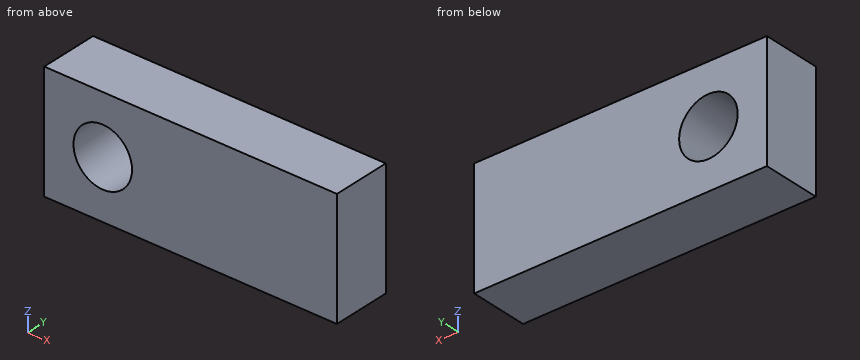
```python
from build123d import *

# Parameters (mm, degrees)
SKETCH2_W           = 127
SKETCH2_H           = 50.8
BOSS_EXTRUDE2_DEPTH = 25.4
CUT_EXTRUDE1_REACH  = 27.4
SKETCH3_R           = 12.7


with BuildPart() as part:
    # Sketch2 → Boss-Extrude2 (new body)
    with BuildSketch(Plane(origin=(0, 0, 0), x_dir=(1, 0, 0), z_dir=(0, 1, 0))):
        with Locations((63.5, 25.4)):
            Rectangle(SKETCH2_W, SKETCH2_H)
    extrude(amount=BOSS_EXTRUDE2_DEPTH)

    # Sketch3 → Cut-Extrude1 (cut, up to next)
    with BuildSketch(Plane.XZ, mode=Mode.PRIVATE) as cut_extrude1_sk1:
        with Locations((25.4, -25.4)):
            Circle(SKETCH3_R)
    cut_extrude1_tool1 = extrude(cut_extrude1_sk1.sketch, amount=-CUT_EXTRUDE1_REACH, mode=Mode.PRIVATE) & part.part
    add(cut_extrude1_tool1.solids().sort_by_distance((25.4, 0, -25.4))[0], mode=Mode.SUBTRACT)


solid = part.part
```
CAD build for the part. Positions are in the model's coordinates, mm. Give positions to 0.01 mm unless a question says otherwise; leave off trailing zeros. Write each loop counter-clockwise with the first axis right and the second up, starting at its lowest first coordinate (ties: lowest second). Pieces come first, ordered by that corner, then holes. Notation, with made-up numbers: (-32.75, 62.5) -> (-24.75, 62.5) arc R23 ccw to (-24.75, 84.5) -> close; hole circle Ø11 at (42.5, 43.5). An arc over 180 degrees is marked (long way). Write each question's results on one line, items separated by ' | '.
1. Cut at A-A, the plane x = 25.4. Write the cut outline in (y, z).
Geometry check:
outline: (0, -50.8) -> (25.4, -50.8) -> (25.4, -38.1) -> (0, -38.1) -> close; (0, -12.7) -> (25.4, -12.7) -> (25.4, 0) -> (0, 0) -> close
2. Cut at C-C, the plane y = 4.75. Write the cut outline in (x, z), then the cut area to 3 significant figures.
Geometry check:
outline: (0, -50.8) -> (127, -50.8) -> (127, 0) -> (0, 0) -> close; hole circle Ø25.4 at (25.4, -25.4) | area: 5,940 mm²
3. Cut at B-B, the plane z = -25.4. Write the cut outline in (x, y).
Geometry check:
outline: (0, 0) -> (12.7, 0) -> (12.7, 25.4) -> (0, 25.4) -> close; (38.1, 0) -> (127, 0) -> (127, 25.4) -> (38.1, 25.4) -> close
4. Wall check: probe 1 along Z at (x, y) = (25.4, 14.25); probe 2 along Z at (x, y) = (31.5, 19.5); probe 3 along X at (y, z) = (22.75, -19). Give the ranges that are in metal, low to high. Write a range as [from, to].
Geometry check:
probe 1: [-50.8, -38.1], [-12.7, 0] | probe 2: [-50.8, -36.54], [-14.26, 0] | probe 3: [0, 14.43], [36.37, 127]
